```python
from build123d import *

# Parameters (mm, degrees)
BOSS_EXTRUDE2_DEPTH     = 7
CUT_EXTRUDE2_DEPTH      = 30.130224853
CUT_EXTRUDE2_DEPTH_BACK = 30.130224853
SKETCH3_R               = 2
BOSS_EXTRUDE3_DEPTH     = 36
SKETCH5_R               = 2
BOSS_EXTRUDE4_DEPTH     = 7
SKETCH14_W              = 49.8
SKETCH14_H              = 5
BOSS_EXTRUDE7_DEPTH     = 30
SKETCH16_W              = 49.8
SKETCH16_H              = 5
BOSS_EXTRUDE8_DEPTH     = 12.25
BOSS_EXTRUDE9_DEPTH     = 5
FILLET1_DEPTH           = 50
FILLET1_2_DEPTH         = 7
FILLET1_START           = 43
FILLET1_3_DEPTH         = 7
FILLET2_R               = 4
FILLET3_R               = 1
CUT_EXTRUDE3_DEPTH      = 191.690493415
CUT_EXTRUDE3_DEPTH_BACK = 191.690493415
SKETCH19_R              = 2.625


with BuildPart() as part:
    # Sketch1 → Boss-Extrude2 (new body)
    with BuildSketch(Plane(origin=(0, 0, 0), x_dir=(1, 0, 0), z_dir=(0, 1, 0))):
        with BuildLine():
            Line((-24.9, 0), (-24.9, 13.4))
            Line((-24.9, 13.4), (24.9, 13.4))
            Line((24.9, 13.4), (24.9, 0))
            ThreePointArc((24.9, 0), (23.392904185, -4.800819919), (19.412411454, -7.878950407))
            Line((19.412411454, -7.878950407), (8.235013612, 1.5))
            ThreePointArc((8.235013612, 1.5), (11.116692467, 6.448255578), (16.5, 8.4))
            Line((16.5, 8.4), (-16.5, 8.4))
            ThreePointArc((-16.5, 8.4), (-11.116692467, 6.448255578), (-8.235013612, 1.5))
            Line((-8.235013612, 1.5), (-19.412411454, -7.878950407))
            ThreePointArc((-19.412411454, -7.878950407), (-23.392904185, -4.800819919), (-24.9, 0))
        make_face()
    extrude(amount=BOSS_EXTRUDE2_DEPTH)

    # Sketch3 → Cut-Extrude2 (cut, two sides: drawn at the far end of the back side and taken through both)
    with BuildSketch(Plane(origin=(0, 7, 0), x_dir=(1, 0, 0), z_dir=(0, 1, 0)).offset(-CUT_EXTRUDE2_DEPTH_BACK)):
        with Locations(Location((-16.5, 0, 0), (0, 0, 270))):
            Circle(SKETCH3_R)
        with Locations(Location((16.5, 0, 0), (0, 0, 270))):
            Circle(SKETCH3_R)
    extrude(amount=CUT_EXTRUDE2_DEPTH + CUT_EXTRUDE2_DEPTH_BACK, mode=Mode.SUBTRACT)

    # Sketch4 → Boss-Extrude3 (add)
    with BuildSketch(Plane(origin=(0, 7, 0), x_dir=(1, 0, 0), z_dir=(0, 1, 0))):
        Polygon((-24.9, 13.4), (-24.9, 0), (-20.9, 0), (-20.9, 8.4), (-16.5, 8.4), (16.5, 8.4), (20.9, 8.4), (20.9, 0), (24.9, 0), (24.9, 13.4), align=None)
    extrude(amount=BOSS_EXTRUDE3_DEPTH)

    # Sketch5 → Boss-Extrude4 (add)
    with BuildSketch(Plane(origin=(0, 43, 0), x_dir=(1, 0, 0), z_dir=(0, 1, 0))):
        with BuildLine():
            Line((-24.9, 13.4), (-24.9, 0))
            ThreePointArc((-24.9, 0), (-23.392904185, -4.800819919), (-19.412411454, -7.878950407))
            Line((-19.412411454, -7.878950407), (-8.235013612, 1.5))
            ThreePointArc((-8.235013612, 1.5), (-11.116692467, 6.448255578), (-16.5, 8.4))
            Line((-16.5, 8.4), (16.5, 8.4))
            ThreePointArc((16.5, 8.4), (11.116692467, 6.448255578), (8.235013612, 1.5))
            Line((8.235013612, 1.5), (19.412411454, -7.878950407))
            ThreePointArc((19.412411454, -7.878950407), (23.392904185, -4.800819919), (24.9, 0))
            Line((24.9, 0), (24.9, 13.4))
            Line((24.9, 13.4), (-24.9, 13.4))
        make_face()
        with Locations(Location((16.5, 0, 0), (0, 0, 270))):
            Circle(SKETCH5_R, mode=Mode.SUBTRACT)
        with Locations(Location((-16.5, 0, 0), (0, 0, 270))):
            Circle(SKETCH5_R, mode=Mode.SUBTRACT)
    extrude(amount=BOSS_EXTRUDE4_DEPTH)

    # Sketch14 → Boss-Extrude7 (add)
    with BuildSketch(Plane(origin=(0, 50, 0), x_dir=(1, 0, 0), z_dir=(0, 1, 0))):
        with Locations((0, 10.9)):
            Rectangle(SKETCH14_W, SKETCH14_H)
    extrude(amount=BOSS_EXTRUDE7_DEPTH)

    # Sketch16 → Boss-Extrude8 (add)
    with BuildSketch(Plane.XZ):
        with Locations((0, -10.9)):
            Rectangle(SKETCH16_W, SKETCH16_H)
    extrude(amount=BOSS_EXTRUDE8_DEPTH)

    # Sketch17 → Boss-Extrude9 (add)
    with BuildSketch(Plane(origin=(0, 0, -13.4), x_dir=(-1, 0, 0), z_dir=(0, 0, -1))):
        Polygon((24.9, 80), (-24.9, 80), (-54.131101944, 73.25146837), (-67.628165204, 131.713672257), (79.608841274, 165.706013609), (93.105904535, 107.243809722), (24.9, 91.497235918), align=None)
    extrude(amount=-BOSS_EXTRUDE9_DEPTH)

    # Fillet1: read off the stored shape, not the designer's step
    # Fillet1 outline → Fillet1 (cut)
    with BuildSketch(Plane(origin=(0, 0, 0), x_dir=(1, 0, 0), z_dir=(0, 1, 0))):
        with BuildLine():
            Line((-19.412411454, -7.878950407), (-17.191978394, -6.015785846))
            ThreePointArc((-17.191978394, -6.015785846), (-20.037614317, -6.942179175), (-22.729609591, -5.63488814))
            ThreePointArc((-22.729609591, -5.63488814), (-21.206707029, -6.957507379), (-19.412411454, -7.878950407))
        make_face()
        with BuildLine():
            ThreePointArc((22.729609591, -5.63488814), (20.037614317, -6.942179175), (17.191978394, -6.015785846))
            Line((17.191978394, -6.015785846), (19.412411454, -7.878950407))
            ThreePointArc((19.412411454, -7.878950407), (21.206707029, -6.957507379), (22.729609591, -5.63488814))
        make_face()
    extrude(amount=FILLET1_DEPTH, mode=Mode.SUBTRACT)

    # Fillet1 2 outline → Fillet1 2 (add)
    with BuildSketch(Plane(origin=(0, 0, 0), x_dir=(1, 0, 0), z_dir=(0, 1, 0))):
        with BuildLine():
            Line((16.5, 8.4), (4.906898603, 8.4))
            ThreePointArc((4.906898603, 8.4), (8.19911817, 6.671847337), (8.646608731, 2.980645161))
            ThreePointArc((8.646608731, 2.980645161), (11.729120592, 6.91366109), (16.5, 8.4))
        make_face()
        with BuildLine():
            ThreePointArc((-16.5, 8.4), (-11.729120592, 6.91366109), (-8.646608731, 2.980645161))
            ThreePointArc((-8.646608731, 2.980645161), (-8.19911817, 6.671847337), (-4.906898603, 8.4))
            Line((-4.906898603, 8.4), (-16.5, 8.4))
        make_face()
    extrude(amount=FILLET1_2_DEPTH)

    # Fillet1 3 outline → Fillet1 3 (add)
    with BuildSketch(Plane(origin=(0, 0, 0), x_dir=(1, 0, 0), z_dir=(0, 1, 0)).offset(FILLET1_START)):
        with BuildLine():
            Line((16.5, 8.4), (4.906898603, 8.4))
            ThreePointArc((4.906898603, 8.4), (8.19911817, 6.671847337), (8.646608731, 2.980645161))
            ThreePointArc((8.646608731, 2.980645161), (11.729120592, 6.91366109), (16.5, 8.4))
        make_face()
        with BuildLine():
            ThreePointArc((-16.5, 8.4), (-11.729120592, 6.91366109), (-8.646608731, 2.980645161))
            ThreePointArc((-8.646608731, 2.980645161), (-8.19911817, 6.671847337), (-4.906898603, 8.4))
            Line((-4.906898603, 8.4), (-16.5, 8.4))
        make_face()
    extrude(amount=FILLET1_3_DEPTH)

    # Fillet2
    fillet2_edges = [part.edges().sort_by_distance(p)[0] for p in [
        (8.235013612, 46.5, -1.5),
        (-8.235013612, 46.5, -1.5),
        (8.235013612, 3.5, -1.5),
        (-8.235013612, 3.5, -1.5),
    ]]
    fillet(fillet2_edges, radius=FILLET2_R)

    # Fillet3
    fillet3_edges = [part.edges().sort_by_distance(p)[0] for p in [
        (-24.9, 25, 0),
        (-20.9, 25, 0),
        (-20.9, 25, -8.4),
        (20.9, 25, -8.4),
        (20.9, 25, 0),
        (24.9, 25, 0),
    ]]
    fillet(fillet3_edges, radius=FILLET3_R)

    # Sketch19 → Cut-Extrude3 (cut, two sides: drawn at the far end of the back side and taken through both)
    with BuildSketch(Plane.XY.offset(-8.4).offset(-CUT_EXTRUDE3_DEPTH_BACK)):
        with Locations((-75.116087748, 118.485094879)):
            Circle(SKETCH19_R)
        with Locations((42.889816787, 91.241285157)):
            Circle(SKETCH19_R)
        with Locations(Location((49.638348417, 120.4723871, 0), (0, 0, 180))):
            Circle(SKETCH19_R)
        with Locations(Location((-68.367556118, 147.716196822, 0), (0, 0, 180))):
            Circle(SKETCH19_R)
    extrude(amount=CUT_EXTRUDE3_DEPTH + CUT_EXTRUDE3_DEPTH_BACK, mode=Mode.SUBTRACT)


solid = part.part
```
Geometry: final body of the model. Coordinates: model frame, mm. A direction names the side the tool comes from. Round coordinates to 2 decimals unless told otherwise and drop trailing zeros. Loops run counter-clockwise (first coordinate to the right, second up) from the corner with the lowest first, then second, coordinate; pieces in that order, holes last. Notation, with made-up numbers: (-3, 42) -> (16, 42) arc R32 cw to (16, 72) -> close; hole circle Ø9 at (22.25, 28). An arc over 180 degrees is marked (long way). Use one line per item in the form item = value. Start each with the question number.
1) Section B-B on x = -69. Output: boundary loops of the cut face in (y, z).
2) Access query for faces 4 (the flat face through (-17, 50, -3)), 5 (the cylindrical face through (7.955, 3.451, -6.991)), 6 (the flat face through (20.9, 25, -4)), 7 (the flat face through (17, 0, -3)), 8 (the flat face through (39.311, 76.673, -10.935)). Directions: +Z, -Z, +X, -X, +Y, -Y. A direction counts if a zero-diameter tool reaches every point of the face in a straight line with its end or side. Return the directions, or none.
3) Section A-A on y = 13. Output: boundary loops of the cut face in (x, z).
4) Draft query along Z for faces 1 (the flat face through (-24.9, 29, -8)), 2 (the cylindrical face through (20.08, 46.45, 6.94)), 3 (the cylindrical face through (18.483, 3.451, -0.26)). Return one class per face: released by +Z, released by -Z, zero draft, split by the parting line, or undercut.
5) First-contact query: P1, Ø3, axis at y = 17, z = -3, coming from the -X side; P2, Ø12, axis at x = -4.5, z = -2.5, coming from the +Y side; P3, Ø8, axis at x = -0.5, y = 140, coming from the +Z side. Flat tips, straight axial feed; report the tip coordinate or a pass-through.
6) Section C-C on x = -34. Output: boundary loops of the cut face in (y, z).
7) Line query: L1, parallel to Y at x = 16.5, z = -7.75; L2, parallel to Z at x = 29, y = 114; L3, parallel to X at y = 71.5, z = -10.25. Output: solid intervals per line, ascending.
8) Section D-D on y = 57. Output: boundary loops of the cut face in (x, z), then the cut area to 3 significant figures.
Response:
q1.outline = (101.68, -13.4) -> (145.17, -13.4) -> (145.17, -8.4) -> (101.68, -8.4) -> close; (150.26, -13.4) -> (163.26, -13.4) -> (163.26, -8.4) -> (150.26, -8.4) -> close
q2.face_4 = +Z, +X, -X, +Y
q2.face_5 = +Y, -Y
q2.face_6 = +Z
q2.face_7 = +Z, +X, -X, -Y
q2.face_8 = +Z, -Z, -Y
q3.outline = (-24.9, -13.4) -> (24.9, -13.4) -> (24.9, -1) arc R1 ccw to (23.9, 0) -> (21.9, 0) arc R1 ccw to (20.9, -1) -> (20.9, -7.4) arc R1 cw to (19.9, -8.4) -> (-19.9, -8.4) arc R1 cw to (-20.9, -7.4) -> (-20.9, -1) arc R1 ccw to (-21.9, 0) -> (-23.9, 0) arc R1 ccw to (-24.9, -1) -> close
q4.face_1 = zero draft
q4.face_2 = released by +Z
q4.face_3 = undercut
q5.P1 = -24.9
q5.P2 = 148.62
q5.P3 = -8.4
q6.outline = (93.6, -13.4) -> (155.18, -13.4) -> (155.18, -8.4) -> (93.6, -8.4) -> close
q7.L1 = 0 to 7, 43 to 50
q7.L2 = -13.4 to -8.4
q7.L3 = -24.9 to 24.9
q8.outline = (-24.9, -13.4) -> (24.9, -13.4) -> (24.9, -8.4) -> (-24.9, -8.4) -> close
q8.area = 249 mm^2
